Source: three-view drawing plus pictorial views. Frame: mm from the lowest corner of the part. A direction names the side the tool comes from. Give positions to 0.01 mm unless a question says otherwise; leave off trailing zeros. Loops run counter-clockwise (first coordinate to the right, second up) from the corner with the lowest first, then second, coordinate; pieces in that order, holes last. Notation, with made-up numbers: (24, 39.25) - (81, 39.25) arc R30 ccw to (81, 64.25) - close; hole circle Ø2 at (-36, -29.75). An arc over 180 degrees is marked (long way). Put each result on its own line as item: value.
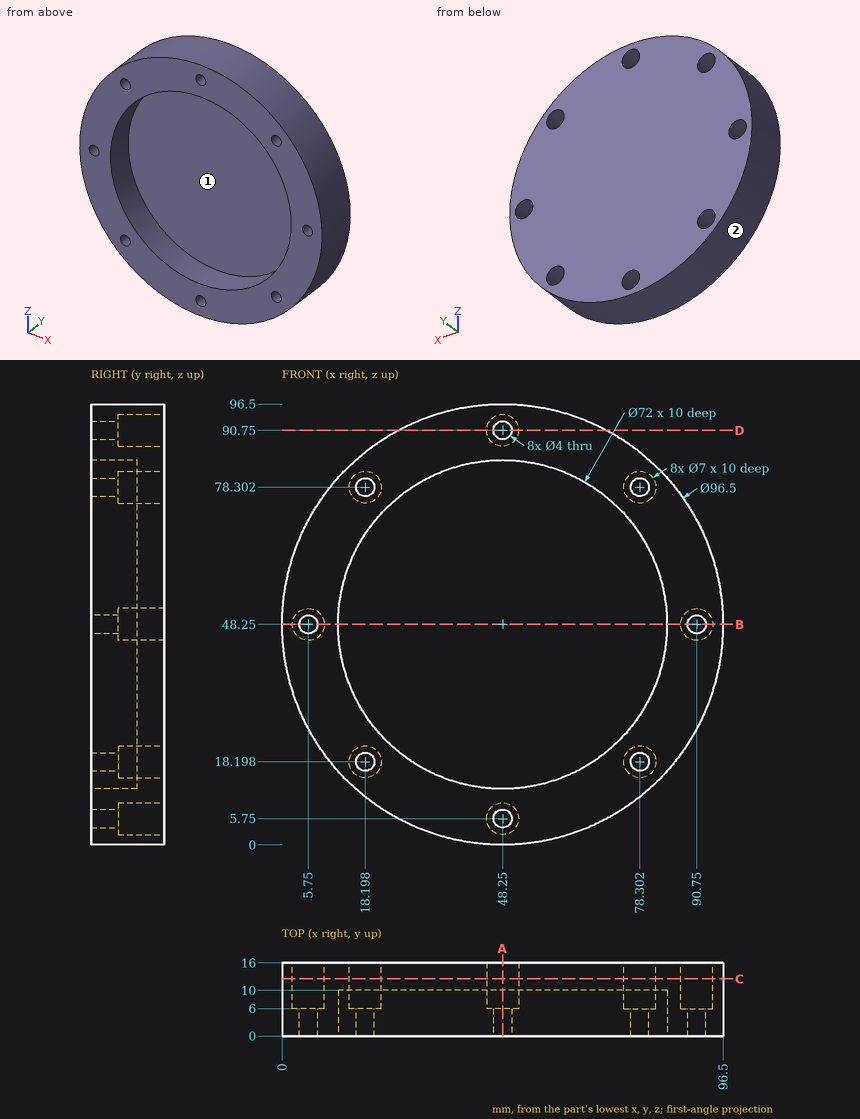
1) Pin query (flat end, axial travel): P1, Ø4, axis at x = 12.5, y = 11.5, coming from the -Z side; P2, Ø8, axis at y = 5.5, z = 21.5, coming from the +X side; P3, Ø6, axis at y = 5.5, z = 77, coming from the +X side. Return the tip coordinate at first contact, or that it passes through.
Check result:
P1: z = 13.77
P2: x = 90.8
P3: x = 89.05
2) Material intervals for line 1 along Z through (x, y) = (47, 5.5); line 2 along Y through (x, z) = (26, 30.5); line 3 along X through (y, z) = (4, 64.5), sorted ascending. Write a range as [from, to].
Check result:
line 1: [0.02, 4.19], [7.31, 12.27], [84.23, 89.19], [92.31, 96.48]
line 2: [10, 16]
line 3: [2.82, 16.13], [80.37, 93.68]
3) Section query B-B, the plane z = 48.25. Output: boundary loops of the cut face in (x, y).
Check result:
outline: (0, 0) - (3.75, 0) - (3.75, 6) - (2.25, 6) - (2.25, 16) - (0, 16) - close; (7.75, 0) - (12.25, 0) - (12.25, 10) - (84.25, 10) - (84.25, 0) - (88.75, 0) - (88.75, 6) - (87.25, 6) - (87.25, 16) - (9.25, 16) - (9.25, 6) - (7.75, 6) - close; (92.75, 0) - (96.5, 0) - (96.5, 16) - (94.25, 16) - (94.25, 6) - (92.75, 6) - close
4) Section query C-C, the plane y = 12.5. State how many separate pieces and enclosed holes the cut face has, plus the area to 3 significant figures.
Check result:
separate pieces: 1
enclosed holes: 8
area: 7,010 mm²
5) Section query A-A, the plane x = 48.25. Output: boundary loops of the cut face in (y, z).
Check result:
outline: (0, 0) - (16, 0) - (16, 2.25) - (6, 2.25) - (6, 3.75) - (0, 3.75) - close; (0, 7.75) - (6, 7.75) - (6, 9.25) - (16, 9.25) - (16, 87.25) - (6, 87.25) - (6, 88.75) - (0, 88.75) - (0, 84.25) - (10, 84.25) - (10, 12.25) - (0, 12.25) - close; (0, 92.75) - (6, 92.75) - (6, 94.25) - (16, 94.25) - (16, 96.5) - (0, 96.5) - close
6) Section query D-D, the plane z = 90.75. Output: boundary loops of the cut face in (x, y).
Check result:
outline: (25.41, 0) - (46.25, 0) - (46.25, 6) - (44.75, 6) - (44.75, 16) - (25.41, 16) - close; (50.25, 0) - (71.09, 0) - (71.09, 16) - (51.75, 16) - (51.75, 6) - (50.25, 6) - close
7) Access query for the marked faces 1 and 2. Directions: +Z, -Z, +X, -X, +Y, -Y. A direction counts if a zero-diameter tool reaches every point of the face in a straight line with its end or side. Return the directions, or none.
Check result:
face 1: -Y
face 2: +Y, -Y
